from build123d import *

# Parameters (mm, degrees)
SKETCH1_W           = 20
SKETCH1_H           = 210
BOSS_EXTRUDE1_DEPTH = 20
SKETCH2_W           = 20
SKETCH2_H           = 22
CUT_EXTRUDE1_DEPTH  = 15
SKETCH3_W           = 20
SKETCH3_H           = 22
CUT_EXTRUDE2_DEPTH  = 15
SKETCH4_W           = 10
SKETCH4_H           = 15
CUT_EXTRUDE3_DEPTH  = 21
SKETCH5_W           = 20
SKETCH5_H           = 32
BOSS_EXTRUDE2_DEPTH = 16
SKETCH6_W           = 28
SKETCH6_H           = 13.5
CUT_EXTRUDE4_DEPTH  = 21


with BuildPart() as part:
    # Sketch1 → Boss-Extrude1 (new body)
    with BuildSketch(Plane(origin=(0, 0, 0), x_dir=(1, 0, 0), z_dir=(0, 1, 0))):
        with Locations((10, 105)):
            Rectangle(SKETCH1_W, SKETCH1_H)
    extrude(amount=BOSS_EXTRUDE1_DEPTH)

    # Sketch2 → Cut-Extrude1 (cut)
    with BuildSketch(Plane(origin=(0, 20, 0), x_dir=(1, 0, 0), z_dir=(0, 1, 0))):
        with Locations((10, 16)):
            Rectangle(SKETCH2_W, SKETCH2_H)
    extrude(amount=-CUT_EXTRUDE1_DEPTH, mode=Mode.SUBTRACT)

    # Sketch3 → Cut-Extrude2 (cut)
    with BuildSketch(Plane(origin=(0, 20, 0), x_dir=(1, 0, 0), z_dir=(0, 1, 0))):
        with Locations((10, 194)):
            Rectangle(SKETCH3_W, SKETCH3_H)
    extrude(amount=-CUT_EXTRUDE2_DEPTH, mode=Mode.SUBTRACT)

    # Sketch4 → Cut-Extrude3 (cut, through all)
    with BuildSketch(Plane(origin=(0, 20, 0), x_dir=(1, 0, 0), z_dir=(0, 1, 0))):
        with Locations((10, 39.5)):
            Rectangle(SKETCH4_W, SKETCH4_H)
        with Locations((10, 64.5)):
            Rectangle(SKETCH4_W, SKETCH4_H)
        with Locations((10, 89.5)):
            Rectangle(SKETCH4_W, SKETCH4_H)
        with Locations((10, 114.5)):
            Rectangle(SKETCH4_W, SKETCH4_H)
        with Locations((10, 139.5)):
            Rectangle(SKETCH4_W, SKETCH4_H)
        with Locations((10, 164.5)):
            Rectangle(SKETCH4_W, SKETCH4_H)
    extrude(amount=-CUT_EXTRUDE3_DEPTH, mode=Mode.SUBTRACT)

    # Sketch5 → Boss-Extrude2 (add)
    with BuildSketch(Plane(origin=(0, 0, 0), x_dir=(-1, 0, 0), z_dir=(0, -1, 0))):
        with Locations((-10, 105)):
            Rectangle(SKETCH5_W, SKETCH5_H)
    extrude(amount=BOSS_EXTRUDE2_DEPTH)

    # Sketch6 → Cut-Extrude4 (cut, through all)
    with BuildSketch(Plane(origin=(20, 0, 0), x_dir=(0, 0, -1), z_dir=(1, 0, 0))):
        with Locations((105, -7.25)):
            Rectangle(SKETCH6_W, SKETCH6_H)
    extrude(amount=-CUT_EXTRUDE4_DEPTH, mode=Mode.SUBTRACT)


solid = part.part
Source: CAD feature listing. Evaluate the final solid. Frame: model axes, mm. A direction names the side the tool comes from. Coordinates: 2 decimals unless noted, no trailing zeros. Loops run counter-clockwise (first coordinate to the right, second up) from the corner with the lowest first, then second, coordinate; pieces in that order, holes last. Notation, with made-up numbers: (88, 0) -> (116, 0) arc R20 ccw to (116, 15) -> close; hole circle Ø8 at (83, -1). An arc over 180 degrees is marked (long way). Answer in a Markdown table with one row per item. Add a question column.
Q1. Section B-B on y = 2.5. Return the cut outline in (x, z), and give its area (3 significant figures).
Q2. Contact query for flat-ended pins moving along their axis: pin 1 Ø10 at (x, z) = (10.5, -185.5) entering from -Y; pin 2 Ø4 at (x, y) = (11, -8) entering from -Z; pin 3 Ø6 at (x, z) = (10.5, -193.5) entering from +Y; pin 4 Ø3 at (y, z) = (-7, -123) entering from -X. Output: stop coordinate, or through.
Q3. Pull-direction query (X, two-part tool) for faces 5 (the face through (10, 0, -93)), 6 (the face through (10, 10, -132)), 7 (the face through (0, 10, -104)), 8 (the face through (10, -16, -105)); classes: pulls with the +X half, pulls with the -X half, needs draft (parallel to the pull), parting line crosses it, or undercut.
Q4. Ray query, line 1 along Z through (x, y) = (2, 17); line 2 along X through (y, z) = (7, -171.5); line 3 along Z through (x, y) = (16.5, -13). Return the intervals inside material, ascending.
Q5. Section A-A on x = 2.5. Return the cut outline in (y, z).
Q6. Section C-C on x = 12. Give the number of separate pieces and of enclosed holes in the cut face, and give its area (3 significant figures).
Q7. Section D-D on z = -189. Return the cut outline in (x, y), and give its area (3 significant figures).
Q8. Reachability of faces 1 (the face through (10, -7, -91)), 2 (the face through (10, -8, -89)), 3 (the face through (5, 10, -139)), 4 (the face through (10, 0, -176)) from +Z, -Z, +X, -X, +Y, -Y: full face, straight path, thin tool, end or side. Return the list, or none.
Computed values:
| question | item | result |
|---|---|---|
| 1 | outline | (0, -210) -> (20, -210) -> (20, 0) -> (0, 0) -> close; hole (5, -172) -> (15, -172) -> (15, -157) -> (5, -157) -> close; hole (5, -147) -> (15, -147) -> (15, -132) -> (5, -132) -> close; hole (5, -122) -> (15, -122) -> (15, -107) -> (5, -107) -> close; hole (5, -97) -> (15, -97) -> (15, -82) -> (5, -82) -> close; hole (5, -72) -> (15, -72) -> (15, -57) -> (5, -57) -> close; hole (5, -47) -> (15, -47) -> (15, -32) -> (5, -32) -> close |
| 1 | area | 3,300 mm^2 |
| 2 | pin 1 | stops at y = 0 |
| 2 | pin 2 | stops at z = -121 |
| 2 | pin 3 | stops at y = 5 |
| 2 | pin 4 | passes through |
| 3 | face 5 | undercut |
| 3 | face 6 | undercut |
| 3 | face 7 | pulls with the -X half |
| 3 | face 8 | needs draft |
| 4 | line 1 | z = -210 to -205, -183 to -27, -5 to 0 |
| 4 | line 2 | x = 0 to 5, 15 to 20 |
| 4 | line 3 | z = -121 to -119, -91 to -89 |
| 5 | outline | (-16, -121) -> (0, -121) -> (0, -210) -> (20, -210) -> (20, -205) -> (5, -205) -> (5, -183) -> (20, -183) -> (20, -27) -> (5, -27) -> (5, -5) -> (20, -5) -> (20, 0) -> (0, 0) -> (0, -89) -> (-16, -89) -> close; hole (-14, -119) -> (-0.5, -119) -> (-0.5, -91) -> (-14, -91) -> close |
| 6 | separate pieces | 7 |
| 6 | enclosed holes | 1 |
| 6 | area | 1,870 mm^2 |
| 7 | outline | (0, 0) -> (20, 0) -> (20, 5) -> (0, 5) -> close |
| 7 | area | 100 mm^2 |
| 8 | face 1 | +X, -X |
| 8 | face 2 | +Z, +X, -X, -Y |
| 8 | face 3 | +Y, -Y |
| 8 | face 4 | -Z, +X, -X, -Y |
